Could you check a few things on this model? Use its own coordinates, in mm. A direction names the side the tool comes from. Give positions to 0.01 mm unless a question says otherwise; leave off trailing zeros. Loops run counter-clockwise (first coordinate to the right, second up) from the corner with the lowest first, then second, coordinate; pieces in that order, holes last. Notation, with made-up numbers: (6, 33) -> (12, 33) arc R20 ccw to (12, 47) -> close; hole circle Ø5 at (61.25, 53.5). An arc over 180 degrees is marked (long way). Put each result on its own line as item: value.
```python
from build123d import *

# Parameters (mm, degrees)
BOSS_EXTRUDE1_DEPTH = 4.064
CUT_EXTRUDE1_DEPTH  = 5.064


with BuildPart() as part:
    # Sketch1 → Boss-Extrude1 (new body)
    with BuildSketch(Plane.XY):
        Polygon((125.750548905, 0), (-105.897451095, 0), (-105.897451095, -31.75), (-109.961451095, -31.75), (-109.961451095, -44.45), (-105.897451095, -44.45), (-105.897451095, -88.9), (-109.961451095, -88.9), (-109.961451095, -101.6), (-105.897451095, -101.6), (-105.897451095, -120.65), (125.750548905, -120.65), (125.750548905, -107.95), (129.814548905, -107.95), (129.814548905, -95.25), (125.750548905, -95.25), (125.750548905, -31.75), (129.814548905, -31.75), (129.814548905, -19.05), (125.750548905, -19.05), align=None)
    extrude(amount=BOSS_EXTRUDE1_DEPTH)

    # Sketch2 → Cut-Extrude1 (cut, through all)
    with BuildSketch(Plane.XY.offset(4.064)):
        with BuildLine():
            Line((-74.147451095, -12.7), (94.000548905, -12.7))
            ThreePointArc((94.000548905, -12.7), (102.980805026, -16.419743879), (106.700548905, -25.4))
            Line((106.700548905, -25.4), (106.700548905, -88.9))
            ThreePointArc((106.700548905, -88.9), (102.980805026, -97.880256121), (94.000548905, -101.6))
            Line((94.000548905, -101.6), (-74.147451095, -101.6))
            ThreePointArc((-74.147451095, -101.6), (-83.127707216, -97.880256121), (-86.847451095, -88.9))
            Line((-86.847451095, -88.9), (-86.847451095, -25.4))
            ThreePointArc((-86.847451095, -25.4), (-83.127707216, -16.419743879), (-74.147451095, -12.7))
        make_face()
    extrude(amount=-CUT_EXTRUDE1_DEPTH, mode=Mode.SUBTRACT)


solid = part.part
```
1. If we section it at C-C (x = -83.5): List the corners of the cut face in (y, z) for me, then the cut area to 3 significant figures.
Recorded:
outline: (-120.65, 0) -> (-97.49, 0) -> (-97.49, 4.06) -> (-120.65, 4.06) -> close; (-16.81, 0) -> (0, 0) -> (0, 4.06) -> (-16.81, 4.06) -> close
area: 162 mm^2
2. For faces 4 (the face through (-105.897, -16, 2)), 5 (the face through (125.751, -114, 2)), 6 (the face through (9, -12.7, 2)), 7 (the face through (128, -95.25, 2)), which set-ups out of +Z, -Z, +X, -X, +Y, -Y let a thin tool reach every point of the face, with its end or its side?
Recorded:
face 4: +Z, -Z, -X, +Y
face 5: +Z, -Z, +X, -Y
face 6: +Z, -Z
face 7: +Z, -Z, +X
3. Thinking about a two-plate mould opening in X: for faces 1 (the face through (102.88, -16.32, 2.06)), 2 (the face through (-109.961, -38, 2)), 3 (the face through (-108, -101.6, 2)), which applies, pulls with the +X half, pulls with the -X half, needs draft (parallel to the pull), parting line crosses it, or undercut?
Recorded:
face 1: undercut
face 2: pulls with the -X half
face 3: needs draft
4. I need wall thicknesses on line 1 (Y direction, x = 22.5, z = 0.7); line 2 (X direction, y = -28.5, z = 3.5); line 3 (X direction, y = -87.5, z = 2.05). Which ranges of each line are inside material? Lowest first, please.
Recorded:
line 1: y = -120.65 to -101.6, -12.7 to 0
line 2: x = -105.9 to -86.85, 106.7 to 129.81
line 3: x = -105.9 to -86.85, 106.7 to 125.75
5. I'm going to push flat-ended pins straight in: pin 1 (1.2 mm diameter, centred on x = 128.5, z = 1.5, fed in from +Y); pin 2 (2 mm diameter, centred on y = -23, z = 2, fed in from -X); pin 3 (1.2 mm diameter, centred on y = -52, z = 2.5, fed in from +X). Where does each tip first touch, or does it pass through?
Recorded:
pin 1: stops at y = -19.05
pin 2: stops at x = -105.9
pin 3: stops at x = 125.75
6. If we section it at B-B (z = 1.8): List the corners of the cut face in (x, y) for me.
Recorded:
outline: (-109.96, -101.6) -> (-105.9, -101.6) -> (-105.9, -120.65) -> (125.75, -120.65) -> (125.75, -107.95) -> (129.81, -107.95) -> (129.81, -95.25) -> (125.75, -95.25) -> (125.75, -31.75) -> (129.81, -31.75) -> (129.81, -19.05) -> (125.75, -19.05) -> (125.75, 0) -> (-105.9, 0) -> (-105.9, -31.75) -> (-109.96, -31.75) -> (-109.96, -44.45) -> (-105.9, -44.45) -> (-105.9, -88.9) -> (-109.96, -88.9) -> close; hole (-86.85, -88.9) arc R12.7 ccw to (-74.15, -101.6) -> (94, -101.6) arc R12.7 ccw to (106.7, -88.9) -> (106.7, -25.4) arc R12.7 ccw to (94, -12.7) -> (-74.15, -12.7) arc R12.7 ccw to (-86.85, -25.4) -> close
7. If we section it at A-A (y = -35): List the corners of the cut face in (x, z) for me.
Recorded:
outline: (-109.96, 0) -> (-86.85, 0) -> (-86.85, 4.06) -> (-109.96, 4.06) -> close; (106.7, 0) -> (125.75, 0) -> (125.75, 4.06) -> (106.7, 4.06) -> close
